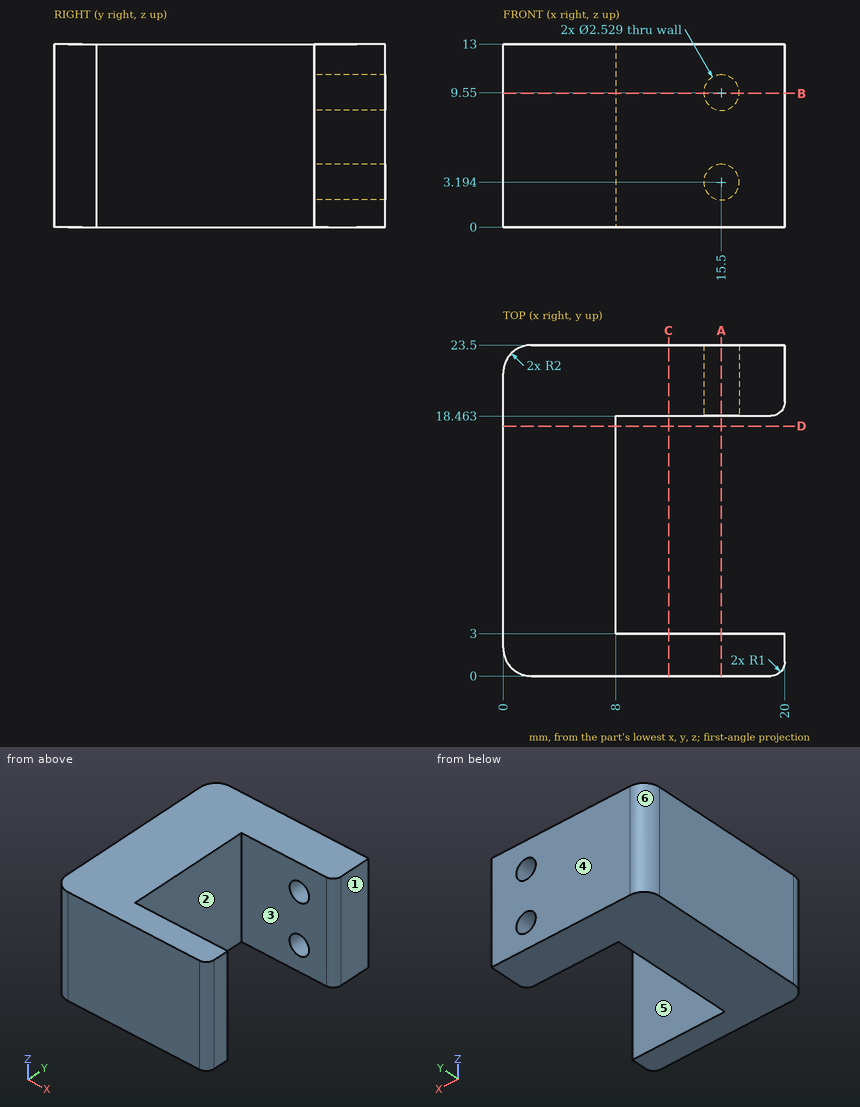
For this review, use the dimensioned drawing (mm, ordinates from the lowest corner) and the shaded views. A direction names the side the tool comes from. Give positions to 0.01 mm unless a question says otherwise; leave off trailing zeros. Loops run counter-clockwise (first coordinate to the right, second up) from the corner with the lowest first, then second, coordinate; pieces in that order, holes last.
Item 1: Take a section at C-C, the plane x = 11.75. State the section outline as (y, z) points.
Item 2: Tool access review of the marked faces 5 and 6: name each direction out of +Z, -Z, +X, -X, +Y, -Y from which nothing blocks a thin tool from reaching the whole face with its end or side.
Item 3: For line 1 along Z through (x, y) = (15.5, 19.55) (1 decimal); line 2 along Y through (x, z) = (18.5, 7.25); line 3 along X through (y, z) = (17.25, 10.75), list the stretches that pass through material, from the lowest coordinate up.
Item 4: Take a section at B-B, the plane z = 9.5. State the section outline as (x, y) points.
Item 5: Take a section at D-D, the plane y = 17.75. State the section outline as (x, z) points, and give its area (3 significant figures).
Item 6: Draft analysis for pull direction Y (two halves, no side actions). For the marked faces 1, 2, 3 and 4, state which applies: +Y half, -Y half, draft (parallel to the pull), parting line (faces both ways), or undercut.
Item 7: Take a section at A-A, the plane x = 15.5. State the section outline as (y, z) points (1 decimal).
Calculated:
1. outline: (0, 0) - (3, 0) - (3, 13) - (0, 13) - close; (18.46, 0) - (23.5, 0) - (23.5, 13) - (18.46, 13) - close
2. face 5: +Z, -Z, +X
2. face 6: +Z, -Z, -X, +Y
3. line 1: z = 0 to 1.9, 4.5 to 8.3, 10.8 to 13
3. line 2: y = 0 to 3, 18.46 to 23.5
3. line 3: x = 0 to 8
4. outline: (0, 2) arc R2 ccw to (2, 0) - (19, 0) arc R1 ccw to (20, 1) - (20, 3) - (8, 3) - (8, 18.46) - (14.24, 18.46) - (14.24, 23.5) - (2, 23.5) arc R2 ccw to (0, 21.5) - close; (16.76, 18.46) - (19, 18.46) arc R1 ccw to (20, 19.46) - (20, 23.5) - (16.76, 23.5) - close
5. outline: (0, 0) - (8, 0) - (8, 13) - (0, 13) - close
5. area: 104 mm2
6. face 1: draft
6. face 2: undercut
6. face 3: undercut
6. face 4: +Y half
7. outline: (0, 0) - (3, 0) - (3, 13) - (0, 13) - close; (18.5, 0) - (23.5, 0) - (23.5, 1.9) - (18.5, 1.9) - close; (18.5, 4.5) - (23.5, 4.5) - (23.5, 8.3) - (18.5, 8.3) - close; (18.5, 10.8) - (23.5, 10.8) - (23.5, 13) - (18.5, 13) - close
